```python
from build123d import *

# Parameters (mm, degrees)
BOSS_EXTRUDE1_DEPTH = 165.1
SKETCH2_R           = 4.25
SKETCH2_R_2         = 6.35
SKETCH2_R_3         = 1.5
CUT_EXTRUDE1_DEPTH  = 11.938
SKETCH3_R           = 2.1
CUT_EXTRUDE2_DEPTH  = 7.874
CUT_EXTRUDE3_DEPTH  = 12.446
SKETCH5_R           = 2.05
CUT_EXTRUDE4_DEPTH  = 6.35
SKETCH6_R           = 2.05
CUT_EXTRUDE5_DEPTH  = 6.35


with BuildPart() as part:
    # Sketch1 → Boss-Extrude1 (new body)
    with BuildSketch(Plane(origin=(0, 0, 0), x_dir=(0, 0, -1), z_dir=(1, 0, 0))):
        with BuildLine():
            Line((-21.9075, -6.6675), (-21.9075, 9.2075))
            Line((-21.9075, 9.2075), (-21.9075, 12.7))
            Line((-21.9075, 12.7), (-25.4, 12.7))
            Line((-25.4, 12.7), (-25.4, -12.7))
            Line((-25.4, -12.7), (25.4, -12.7))
            Line((25.4, -12.7), (25.4, 12.7))
            Line((25.4, 12.7), (21.9075, 12.7))
            Line((21.9075, 12.7), (21.9075, 9.2075))
            Line((21.9075, 9.2075), (21.9075, -6.6675))
            ThreePointArc((21.9075, -6.6675), (21.163551224, -8.463551224), (19.3675, -9.2075))
            Line((19.3675, -9.2075), (-19.3675, -9.2075))
            ThreePointArc((-19.3675, -9.2075), (-21.163551224, -8.463551224), (-21.9075, -6.6675))
        make_face()
    extrude(amount=BOSS_EXTRUDE1_DEPTH)

    # Sketch2 → Cut-Extrude1 (cut)
    with BuildSketch(Plane.XZ.offset(12.7)):
        with Locations(Location((19.05, 0, 0), (0, 0, 270))):
            Circle(SKETCH2_R)
        with Locations(Location((146.05, 0, 0), (0, 0, 270))):
            Circle(SKETCH2_R_2)
        with Locations(Location((19.05, 8.5, 0), (0, 0, 270))):
            Circle(SKETCH2_R_3)
        with Locations(Location((19.05, -8.5, 0), (0, 0, 270))):
            Circle(SKETCH2_R_3)
        with Locations(Location((82.55, 0, 0), (0, 0, 270))):
            Circle(SKETCH2_R_2)
    extrude(amount=-CUT_EXTRUDE1_DEPTH, mode=Mode.SUBTRACT)

    # Sketch3 → Cut-Extrude2 (cut)
    with BuildSketch(Plane.XZ.offset(12.7)):
        with BuildLine():
            Line((52.9, 16.397413762), (52.9, 19.572413762))
            ThreePointArc((52.9, 19.572413762), (50.8, 21.672413762), (48.7, 19.572413762))
            Line((48.7, 19.572413762), (48.7, 16.397413762))
            ThreePointArc((48.7, 16.397413762), (50.8, 18.497413762), (52.9, 16.397413762))
        make_face()
        with Locations((50.8, 16.397413762)):
            Circle(SKETCH3_R)
        with BuildLine():
            Line((52.9, 13.222413762), (52.9, 16.397413762))
            ThreePointArc((52.9, 16.397413762), (50.8, 14.297413762), (48.7, 16.397413762))
            Line((48.7, 16.397413762), (48.7, 13.222413762))
            ThreePointArc((48.7, 13.222413762), (50.8, 11.122413762), (52.9, 13.222413762))
        make_face()
        with BuildLine():
            ThreePointArc((116.4, 13.222413762), (114.3, 11.122413762), (112.2, 13.222413762))
            Line((112.2, 13.222413762), (112.2, 19.572413762))
            ThreePointArc((112.2, 19.572413762), (114.3, 21.672413762), (116.4, 19.572413762))
            Line((116.4, 19.572413762), (116.4, 13.222413762))
        make_face()
        with BuildLine():
            Line((52.9, -19.572413762), (52.9, -13.222413762))
            ThreePointArc((52.9, -13.222413762), (50.8, -11.122413762), (48.7, -13.222413762))
            Line((48.7, -13.222413762), (48.7, -19.572413762))
            ThreePointArc((48.7, -19.572413762), (50.8, -21.672413762), (52.9, -19.572413762))
        make_face()
        with BuildLine():
            Line((112.2, -19.572413762), (112.2, -13.222413762))
            ThreePointArc((112.2, -13.222413762), (114.3, -11.122413762), (116.4, -13.222413762))
            Line((116.4, -13.222413762), (116.4, -19.572413762))
            ThreePointArc((116.4, -19.572413762), (114.3, -21.672413762), (112.2, -19.572413762))
        make_face()
    extrude(amount=-CUT_EXTRUDE2_DEPTH, mode=Mode.SUBTRACT)

    # Sketch4 → Cut-Extrude3 (cut)
    with BuildSketch(Plane.XY.offset(25.4)):
        with BuildLine():
            ThreePointArc((76.2, 12.7), (78.053929045, 8.21582271), (82.533179833, 6.350022277))
            Line((82.533179833, 6.350022277), (82.536543857, 12.7))
            Line((82.536543857, 12.7), (76.2, 12.7))
        make_face()
        with BuildLine():
            Line((82.536543857, 12.7), (82.533179833, 6.350022277))
            ThreePointArc((82.533179833, 6.350022277), (87.03417729, 8.203929045), (88.9, 12.7))
            Line((88.9, 12.7), (82.536543857, 12.7))
        make_face()
        with BuildLine():
            Line((76.2, 12.7), (82.536543857, 12.7))
            Line((82.536543857, 12.7), (82.539907889, 19.04999198))
            ThreePointArc((82.539907889, 19.04999198), (78.056305256, 17.186558542), (76.2, 12.7))
        make_face()
        with BuildLine():
            Line((82.539907889, 19.04999198), (82.536543857, 12.7))
            Line((82.536543857, 12.7), (88.9, 12.7))
            ThreePointArc((88.9, 12.7), (87.036558542, 17.193694744), (82.539907889, 19.04999198))
        make_face()
    extrude(amount=-CUT_EXTRUDE3_DEPTH, mode=Mode.SUBTRACT)

    # Sketch5 → Cut-Extrude4 (cut)
    with BuildSketch(Plane.XZ.offset(12.7)):
        with Locations(Location((6.35, 17.78, 0), (0, 0, 270))):
            Circle(SKETCH5_R)
        with Locations(Location((6.35, -17.78, 0), (0, 0, 270))):
            Circle(SKETCH5_R)
        with Locations(Location((82.55, -17.78, 0), (0, 0, 270))):
            Circle(SKETCH5_R)
        with Locations(Location((158.75, -17.78, 0), (0, 0, 270))):
            Circle(SKETCH5_R)
        with Locations(Location((82.55, 17.78, 0), (0, 0, 270))):
            Circle(SKETCH5_R)
        with Locations(Location((158.75, 17.78, 0), (0, 0, 270))):
            Circle(SKETCH5_R)
    extrude(amount=-CUT_EXTRUDE4_DEPTH, mode=Mode.SUBTRACT)

    # Sketch6 → Cut-Extrude5 (cut)
    with BuildSketch(Plane.XY.offset(25.4)):
        with Locations((101.6, -6.35)):
            Circle(SKETCH6_R)
        with Locations((63.5, -6.35)):
            Circle(SKETCH6_R)
    extrude(amount=-CUT_EXTRUDE5_DEPTH, mode=Mode.SUBTRACT)


solid = part.part
```
Could you check a few things on this model? Use its own coordinates, in mm. A direction names the side the tool comes from. Round coordinates to 2 decimals unless told otherwise and drop trailing zeros. Loops run counter-clockwise (first coordinate to the right, second up) from the corner with the lowest first, then second, coordinate; pieces in that order, holes last. Notation, with made-up numbers: (48, 45) - (92, 45) arc R10 cw to (92, 57) - close; hole circle Ø8 at (23.25, 55). An arc over 180 degrees is marked (long way). Answer in a Markdown table with one row per item. Add a question column.
(1) If we mould it in two halves opening along Z, with no side actions, what happens to faces 1 (the face through (165.1, -10, 0)), 2 (the face through (112.2, -11, -16)), 3 (the face through (81, 0, 25.4)), 4 (the face through (116.4, -11, 16))? For each: pulls with the +Z half, pulls with the -Z half, needs draft (parallel to the pull), parting line crosses it, or undercut.
(2) I'm going to push flat-ended pins straight in: pin 1 (3.5 mm diameter, centred on x = 6.35, z = -17.78, fed in from +Y); pin 2 (3 mm diameter, centred on x = 106, z = 11.5, fed in from +Y). Where does each tip first touch, or does it pass through?
(3) If we section it at B-B (y = -0.5): Please give me the cut outline in (x, z).
(4) I need wall thicknesses on line 1 along Z through (x, y) = (158.75, -10.3); line 2 along X through (y, z) = (-6.35, 23.85); line 3 along X through (y, z) = (-11.65, -17.78). Which ranges of each line are inside material? Lowest first, please.
(5) If we section it at C-C (z = -8.5): Please give me the cut outline in (x, y).
(6) If we section it at D-D (x = 50.8): Please give me the cut outline in (y, z), plus the area to 3 significant figures.
(7) For faces 5 (the face through (0, -10, 0)), 6 (the face through (52.9, -11, 16)), 7 (the face through (81, 3, -21.908)), which set-ups out of +Z, -Z, +X, -X, +Y, -Y let a thin tool reach every point of the face, with its end or its side?
(8) If we section it at A-A (x = 101.6): Please give me the cut outline in (y, z).
Model answer:
| question | item | result |
|---|---|---|
| 1 | face 1 | needs draft |
| 1 | face 2 | undercut |
| 1 | face 3 | pulls with the +Z half |
| 1 | face 4 | undercut |
| 2 | pin 1 | passes through |
| 2 | pin 2 | stops at y = -9.21 |
| 3 | outline | (0, -25.4) - (165.1, -25.4) - (165.1, -21.91) - (0, -21.91) - close; (0, 21.91) - (165.1, 21.91) - (165.1, 25.4) - (0, 25.4) - close |
| 4 | line 1 | z = -25.4 to -19.83, -15.73 to 15.73, 19.83 to 25.4 |
| 4 | line 2 | x = 0 to 61.45, 65.55 to 99.55, 103.65 to 165.1 |
| 4 | line 3 | x = 0 to 4.3, 8.4 to 48.7, 52.9 to 80.5, 84.6 to 112.2, 116.4 to 156.7, 160.8 to 165.1 |
| 5 | outline | (0, -12.7) - (17.55, -12.7) - (17.55, -9.21) - (0, -9.21) - close; (20.55, -12.7) - (165.1, -12.7) - (165.1, -9.21) - (20.55, -9.21) - close |
| 6 | outline | (-12.7, -25.4) - (12.7, -25.4) - (12.7, -21.91) - (-6.67, -21.91) arc R2.54 cw to (-7.73, -21.67) - (-12.7, -21.67) - close; (-12.7, -11.12) - (-9.21, -11.12) - (-9.21, 11.12) - (-12.7, 11.12) - close; (-12.7, 21.67) - (-7.73, 21.67) arc R2.54 cw to (-6.67, 21.91) - (12.7, 21.91) - (12.7, 25.4) - (-12.7, 25.4) - close |
| 6 | area | 258 mm² |
| 7 | face 5 | +Z, -Z, -X, +Y, -Y |
| 7 | face 6 | +Y, -Y |
| 7 | face 7 | +X, -X, +Y |
| 8 | outline | (-12.7, -25.4) - (12.7, -25.4) - (12.7, -21.91) - (-6.67, -21.91) arc R2.54 cw to (-9.21, -19.37) - (-9.21, 19.37) arc R2.54 cw to (-8.4, 21.22) - (-8.4, 25.4) - (-12.7, 25.4) - close; (-4.3, 21.91) - (12.7, 21.91) - (12.7, 25.4) - (-4.3, 25.4) - close |
